Input: part model. Units: mm. Frame: model coordinates. Face numbers are marked on the shaded views. A direction names the side the tool comes from. Give positions to 0.01 mm unless a question says otherwise; leave off trailing zeros. Order: outer loops, then holes, each group sorted by start corner. A loop starts at its lowest first (then second) coordinate and runs counter-clockwise, first axis right, second up. Notation, with made-up numbers: M -14.5,50 L 30.5,50 A33 cw 30.5,87 Z; hole C 30.25,18 d3. An arc over 180 degrees is marked long. Use a Markdown table: item, result.
from build123d import *

# Parameters (mm, degrees)
F0_W      = 31.75
F0_H      = 67.31
F1_DEPTH  = 3.175
F3_DEPTH  = 25.4
F12_W     = 3.175
F12_H     = 0.1778
F14_DEPTH = 0.1778
F15_W     = 31.75
F15_H     = 15.875
F16_DEPTH = 12.7
F15_H_2   = 14.3002
F17_DEPTH = 6.35


with BuildPart() as f1:
    # F0 (on Front) → F1 (new body)
    with BuildSketch(Plane.XZ):
        with Locations((15.875, 33.655)):
            Rectangle(F0_W, F0_H)
        Polygon((31.75, 72.39), (0, 67.31), (31.75, 67.31), align=None)
        Polygon((31.75, 0), (0, 0), (0, -5.08), align=None)
    extrude(amount=F1_DEPTH)

    # F2 (on face) → F3 (cut)
    with BuildSketch(Plane.XZ.offset(3.175)):
        Polygon((0, -2.3622), (0, -2.54), (2.54, -2.54), (2.54, -4.6736), (2.7178, -4.645152), (2.7178, -2.3622), align=None)
        Polygon((2.54, -4.6736), (0, -5.08), (2.54, -5.08), align=None)
        Polygon((0, -2.54), (0, -5.08), (2.54, -4.6736), (2.54, -2.54), align=None)
    extrude(amount=-F3_DEPTH, mode=Mode.SUBTRACT)

    # F5: sweep along a path in F5_path
    with BuildLine(Plane(origin=(31.75, -3.175, 0), x_dir=(0.9874406319, 0, 0.1579905011), z_dir=(0.1579905011, 0, -0.9874406319))) as f5_path:
        Line((0, 0), (-29.4014638061, 0))
    # F4 (on face) → F5 (sweep)
    with BuildSketch(Plane(origin=(2.7178, 0, 0), x_dir=(0, -1, 0), z_dir=(-1, 0, 0))):
        Polygon((0, -5.661152), (3.175, -4.645152), (0, -4.645152), align=None)
    sweep(path=f5_path.line)

    # F7: sweep along a path in F7_path
    with BuildLine(Plane(origin=(31.75, -3.175, 72.39), x_dir=(0.9874406319, 0, 0.1579905011), z_dir=(0.1579905011, 0, -0.9874406319))) as f7_path:
        Line((0, 0), (-32.153831809, 0))
    # F6 (on face) → F7 (sweep)
    with BuildSketch(Plane(origin=(0, 0, 0), x_dir=(0, -1, 0), z_dir=(-1, 0, 0))):
        Polygon((0, 68.326), (0, 67.31), (3.175, 67.31), align=None)
    sweep(path=f7_path.line)

    # F9: sweep along a path in F9_path
    with BuildLine(Plane(origin=(0, -3.175, 67.31), x_dir=(-0.9874406319, 0, -0.1579905011), z_dir=(-0.1579905011, 0, 0.9874406319))) as f9_path:
        Line((0, 0), (-32.153831809, 0))
    # F8 (on face) → F9 (sweep, cut)
    with BuildSketch(Plane.YZ.offset(31.75)):
        Polygon((0, 73.406), (-3.175, 72.39), (-3.175, 72.2122), (0, 73.2282), align=None)
    sweep(path=f9_path.line, mode=Mode.SUBTRACT)

    # F11: sweep along a path in F11_path
    with BuildLine(Plane(origin=(31.75, -3.175, 0), x_dir=(0.9874406319, 0, 0.1579905011), z_dir=(0.1579905011, 0, -0.9874406319))) as f11_path:
        Line((0, 0), (-29.4014638061, 0))
    # F10 (on face) → F11 (sweep, cut)
    with BuildSketch(Plane.YZ.offset(31.75)):
        Polygon((-3.175, 0.1778), (-3.175, 0), (0, -1.016), (0, -0.8382), align=None)
    sweep(path=f11_path.line, mode=Mode.SUBTRACT)

    # F13: sweep along a path in F13_path
    with BuildLine(Plane(origin=(2.7178, 0, -2.3622), x_dir=(0, 0, -1), z_dir=(0, 1, 0))) as f13_path:
        Line((3.121152, 0), (0, 0))
        Line((0, 0), (0, 2.7178))
    # F12 (on face) → F13 (sweep, cut)
    with BuildSketch(Plane(origin=(0, 0, 0), x_dir=(0, -1, 0), z_dir=(-1, 0, 0))):
        with Locations((1.5875, -2.2733)):
            Rectangle(F12_W, F12_H)
    sweep(path=f13_path.line, transition=Transition.RIGHT, mode=Mode.SUBTRACT)

    # F14 (cut): a face of the model
    f14_faces = [f1.faces().sort_by_distance(p)[0] for p in [
        (15.9376220602, 0, 33.8178143866),
    ]]
    extrude(f14_faces, amount=-F14_DEPTH, mode=Mode.SUBTRACT)

    # F15 (on face) → F16 (join)
    with BuildSketch(Plane.XZ.offset(3.175)):
        with Locations((15.875, 44.1325)):
            Rectangle(F15_W, F15_H)
        with Locations((15.875, 28.2575)):
            Rectangle(F15_W, F15_H)
    extrude(amount=F16_DEPTH)

    # F15 (on face) → F17 (join)
    with BuildSketch(Plane.XZ.offset(3.175)):
        with Locations((15.875, 59.2201)):
            Rectangle(F15_W, F15_H_2)
        with Locations((15.875, 13.1699)):
            Rectangle(F15_W, F15_H_2)
    extrude(amount=F17_DEPTH)


solid = f1.part
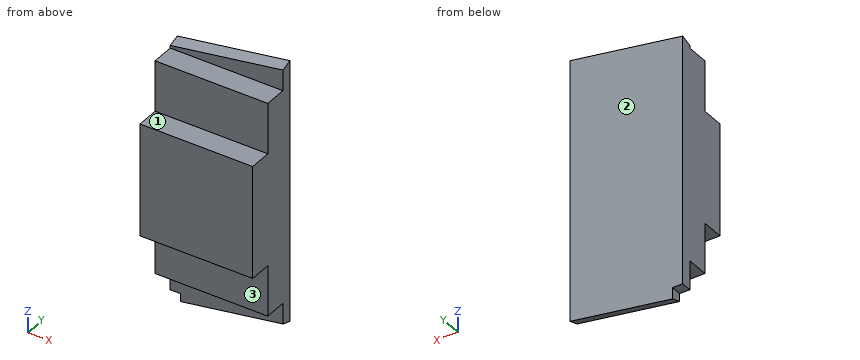
1) First-contact query: pin 1 Ø5 at (y, z) = (-10, 3) entering from +X; pin 2 Ø1.9 at (x, y) = (13, -12) entering from +Z; pin 3 Ø6 at (x, y) = (17.5, -7.5) entering from -Z; pin 4 Ø5 at (x, z) = (10.5, -1.5) entering from -Y (3 decimals). Flat tips, straight axial feed; report the tip coordinate or a pass-through.
Response values:
| item | result |
|---|---|
| pin 1 | passes through |
| pin 2 | stops at z = 52.07 |
| pin 3 | stops at z = 6.02 |
| pin 4 | stops at y = -3.175 |
2) Cut plane C-C on z = 10. Return loops of the section in (x, y) (3 decimals), and give its area (3 significant figures).
Response values:
| item | result |
|---|---|
| outline | M 0,-9.525 L 31.75,-9.525 L 31.75,-0.178 L 0,-0.178 Z |
| area | 297 mm² |
3) Cut plane D-D on x = 2. Return loops of the section in (y, z) (3 decimals), and give its area (3 significant figures).
Response values:
| item | result |
|---|---|
| outline | M -15.875,20.32 L -9.525,20.32 L -9.525,6.02 L -3.175,6.02 L -3.175,-2.184 L -0.178,-2.184 L -0.178,68.411 L -3.175,67.452 L -3.175,66.37 L -9.525,66.37 L -9.525,52.07 L -15.875,52.07 Z |
| area | 795 mm² |
4) Cut plane A-A on x = 25. Return loops of the section in (y, z) (3 decimals).
Response values:
| item | result |
|---|---|
| outline | M -15.875,20.32 L -9.525,20.32 L -9.525,6.02 L -3.175,6.02 L -3.175,-0.902 L -0.178,-1.861 L -0.178,72.091 L -3.175,71.132 L -3.175,66.37 L -9.525,66.37 L -9.525,52.07 L -15.875,52.07 Z |
5) Cut plane B-B on y = -8.5. Return loops of the section in (x, z).
Response values:
| item | result |
|---|---|
| outline | M 0,6.02 L 31.75,6.02 L 31.75,66.37 L 0,66.37 Z |
6) Reachability of the marked faces 1, 2 and 3 from +Z, -Z, +X, -X, +Y, -Y: full face, straight path, thin tool, end or side. Return the list, or none.
Response values:
| item | result |
|---|---|
| face 1 | +Z, +X, -X, -Y |
| face 2 | +Z, -Z, +X, -X, +Y |
| face 3 | -Z, +X, -X, -Y |
7) Material intervals for line 1 (Y direction, x = 27, z = 66) (3 decimals); line 2 (Z direction, x = 8.5, y = -11.5); line 3 (Z direction, x = 25.5, y = -9.25), sorted ascending. Write a range as from..to.
Response values:
| item | result |
|---|---|
| line 1 | y = -9.525..-0.178 |
| line 2 | z = 20.32..52.07 |
| line 3 | z = 6.02..66.37 |
